Part model, mm, in its own coordinate system. A direction names the side the tool comes from. Coordinates: 2 decimals unless noted, no trailing zeros. Write each loop counter-clockwise with the first axis right and the second up, starting at its lowest first coordinate (ties: lowest second). Pieces come first, ordered by that corner, then holes. Notation, with made-up numbers: (-0.75, -3.5) - (58.25, -3.5) arc R24 cw to (58.25, 15.5) - close; hole circle Ø9 at (-29.75, 16). An arc over 180 degrees is marked (long way). Write each question's results on one line, items separated by ' | '.
from build123d import *

# Parameters (mm, degrees)
F0_R     = 17.5
F1_DEPTH = 2
F3_DEPTH = 20
F4_DEPTH = 6.001
F5_DEPTH = 6.001
F6_R     = 5
F7_R     = 0.99999
F8_R     = 0.5


# Not quite as in the source:
# - a fillet or chamfer is up to 0.001 mm smaller than in the source, because OpenCascade refuses the exact size


with BuildPart() as f1:
    # F0 (on Top) → F1 (new body)
    with BuildSketch(Plane.XY):
        Circle(F0_R)
    extrude(amount=F1_DEPTH)

    # F2 (on Front) → F3 (join, symmetric)
    with BuildSketch(Plane.XZ):
        Polygon((-6.75, 8), (-6.75, 2), (6.75, 2), (6.75, 8), (4.75, 8), (4.75, 5), (-4.75, 3), (-4.75, 8), align=None)
    extrude(amount=F3_DEPTH, both=True)

    # F4 (cut, through all): a face of the model
    f4_faces = [f1.faces().sort_by_distance(p)[0] for p in [
        (0, -18.5005607704, 2),
    ]]
    extrude(f4_faces, amount=-F4_DEPTH, mode=Mode.SUBTRACT)

    # F5 (cut, through all): a face of the model
    f5_faces = [f1.faces().sort_by_distance(p)[0] for p in [
        (0, 18.5005607704, 2),
    ]]
    extrude(f5_faces, amount=-F5_DEPTH, mode=Mode.SUBTRACT)

    # F6
    f6_edges = [f1.edges().sort_by_distance(p)[0] for p in [
        (-6.75, 0, 2),
        (6.75, 0, 2),
    ]]
    fillet(f6_edges, radius=F6_R)

    # F7 (radius 1 in the source; OpenCascade refuses exactly that, so slightly less here)
    f7_edges = [f1.edges().sort_by_distance(p)[0] for p in [
        (-6.75, 0, 8),
        (6.75, 0, 8),
    ]]
    fillet(f7_edges, radius=F7_R)

    # F8
    f8_edges = [f1.edges().sort_by_distance(p)[0] for p in [
        (-17.5, 0, 0),
    ]]
    fillet(f8_edges, radius=F8_R)


solid = f1.part
(1) Flat gauge pins, fed straight in: P1, Ø4.5, axis at x = -14, y = 1, coming from the +Z side; P2, Ø4, axis at x = 3.5, z = 6.5, coming from the -Y side; P3, Ø1, axis at x = 0.5, z = 4.5, coming from the +Y side. Where does each tip first touch, or does it go through?
Return value:
P1: stops at z = 2 | P2: stops at y = -17.26 | P3: stops at y = 17.5
(2) 3-axis set-ups, long thin cutter, end or side, ignore diameter. For faces 1 (the flat face through (4.75, 0, 7)), 2 (the flat face through (-5, 0, 8)), 3 (the flat face through (14, 0, 2)): which of +Z, -Z, +X, -X, +Y, -Y reach the whole face in a straight line?
Return value:
face 1: +Z, +Y, -Y | face 2: +Z, +X, -X, +Y, -Y | face 3: +Z, +X, +Y, -Y
(3) Saw through at C-C on x = 0. Write the cut outline in (y, z).
Return value:
outline: (-17.5, 0.5) arc R0.5 ccw to (-17, 0) - (17, 0) arc R0.5 ccw to (17.5, 0.5) - (17.5, 4) - (-17.5, 4) - close
(4) Saw through at D-D on z = 7.5. Write the cut outline in (x, y).
Return value:
outline: (-6.62, -16.2) arc R17.5 ccw to (-4.75, -16.84) - (-4.75, 16.84) arc R17.5 ccw to (-6.62, 16.2) - close; (4.75, -16.84) arc R17.5 ccw to (6.62, -16.2) - (6.62, 16.2) arc R17.5 ccw to (4.75, 16.84) - close
(5) Saw through at A-A on z = 5.5. Write the cut outline in (x, y), then the cut area to 3 significant figures.
Return value:
outline: (-6.98, -16.05) arc R17.5 ccw to (-4.75, -16.84) - (-4.75, 16.84) arc R17.5 ccw to (-6.98, 16.05) - close; (4.75, -16.84) arc R17.5 ccw to (6.98, -16.05) - (6.98, 16.05) arc R17.5 ccw to (4.75, 16.84) - close | area: 147 mm^2
(6) Two-plate mould, pull along X, no slides. Class faces 4 (the cylindrical face through (8.18, -0.23, 3.5)), 5 (the flat face through (-4.75, 0, 5)), 6 (the flat face through (-14, 0, 2)), 7 (the cylindrical face through (-8.18, -0.23, 3.5)): released by +X, released by -X, zero draft, split by the parting line, or undercut.
Return value:
face 4: released by +X | face 5: undercut | face 6: zero draft | face 7: released by -X
(7) Wall check: line 1 (X direction, y = -13, z = 6.75); line 2 (Z direction, x = 12, y = -7); line 3 (X direction, y = 4, z = 7.75). Give the ranges that are in metal, low to high. Write a range as from..to.
Return value:
line 1: x = -6.76..-4.75, 4.75..6.76 | line 2: z = 0..2 | line 3: x = -6.41..-4.75, 4.75..6.41
